Could you check a few things on this model? Use its own coordinates, in mm. Face numbers are marked on the shaded views. A direction names the side the tool comes from. Round coordinates to 2 decimals unless told otherwise and drop trailing zeros. Loops run counter-clockwise (first coordinate to the right, second up) from the corner with the lowest first, then second, coordinate; pieces in that order, holes last. Notation, with made-up numbers: (-23, 4.25) -> (17, 4.25) arc R17 ccw to (17, 30.25) -> close; hole circle Ø8 at (-23.75, -25). An arc over 180 degrees is marked (long way). Put each result on its own line as item: value. Start each with the question number.
1. I'm going to push flat-ended pins straight in: P1, Ø5.5, axis at y = 16, z = -4.5, coming from the +X side; P2, Ø5, axis at x = 6, z = -24.5, coming from the -Y side; P3, Ø8, axis at x = 8, z = -17.5, coming from the +Y side. Where does each tip first touch, or does it pass through?
2. Imagine slicing it at D-D, the plane z = -23.5. Please give me the cut outline in (x, y), and give its area (3 significant figures).
3. Imagine slicing it at C-C, the plane y = 13.5. Please give me the cut outline in (x, z), and give its area (3 significant figures).
4. Which directions (+Z, -Z, +X, -X, +Y, -Y) give clear straight access to the entire face, cutting with the end or side of a thin tool? Please do the marked faces 1, 2 and 3.
5. If we mould it in two halves opening along Y, with no side actions, what happens to the marked faces 4, 5, 6 and 7? For each: pulls with the +Y half, pulls with the -Y half, needs draft (parallel to the pull), parting line crosses it, or undercut.
6. Imagine slicing it at B-B, the plane z = -4. Please give me the cut outline in (x, y), and give its area (3 significant figures).
7. Imagine slicing it at A-A, the plane x = 14.5. Count the separate pieces of the cut face and the enclosed holes in it, and give its area (3 significant figures).
8. I need wall thicknesses on line 1 (Z direction, x = 14.5, y = -0.5); line 2 (X direction, y = -0.5, z = -34); line 3 (Y direction, x = 17, z = -31). Which ranges of each line are inside material? Lowest first, please. Write a range as [from, to].
```python
from build123d import *

# Parameters (mm, degrees)
SALIENTE_EXTRUIR1_DEPTH = 30
REDONDEO1_R             = 1.5
SALIENTE_EXTRUIR2_START = 2.1
SALIENTE_EXTRUIR2_DEPTH = 2.1
SALIENTE_EXTRUIR3_START = 2.1
SALIENTE_EXTRUIR3_DEPTH = 2.1
CROQUIS4_W              = 13.5
CROQUIS4_H              = 8
CROQUIS4_R              = 1.25
SALIENTE_EXTRUIR4_DEPTH = 1
SALIENTE_EXTRUIR5_START = 1
CROQUIS5_W              = 13.5
CROQUIS5_H              = 8
CROQUIS5_R              = 1.25
SALIENTE_EXTRUIR5_DEPTH = 1
REDONDEO2_R             = 1


with BuildPart() as part:
    # Croquis1 → Saliente-Extruir1 (new body)
    with BuildSketch(Plane(origin=(0, 0, 0), x_dir=(1, 0, 0), z_dir=(0, 1, 0))):
        Polygon((0, 0), (9.5, 0), (9.5, 8), (5, 8), (5, 30), (9.5, 30), (9.5, 38), (0, 38), align=None)
    extrude(amount=SALIENTE_EXTRUIR1_DEPTH)

    # Redondeo1
    redondeo1_edges = [part.edges().sort_by_distance(p)[0] for p in [
        (0, 15, -38),
        (9.5, 15, -38),
        (9.5, 15, -30),
        (5, 15, -30),
        (5, 15, -8),
        (9.5, 15, -8),
        (9.5, 15, 0),
        (0, 15, 0),
    ]]
    fillet(redondeo1_edges, radius=REDONDEO1_R)

    # Croquis2 → Saliente-Extruir2 (add)
    with BuildSketch(Plane(origin=(0, 30, 0), x_dir=(1, 0, 0), z_dir=(0, 1, 0)).offset(SALIENTE_EXTRUIR2_START)):
        with BuildLine():
            Line((0, 36.5), (0, 1.5))
            ThreePointArc((0, 1.5), (0.439339828, 0.439339828), (1.5, 0))
            Line((1.5, 0), (8, 0))
            ThreePointArc((8, 0), (9.060660172, 0.439339828), (9.5, 1.5))
            Line((9.5, 1.5), (9.5, 3))
            Line((9.5, 3), (3, 3))
            Line((3, 3), (3, 35))
            Line((3, 35), (9.5, 35))
            Line((9.5, 35), (9.5, 36.5))
            ThreePointArc((9.5, 36.5), (9.060660172, 37.560660172), (8, 38))
            Line((8, 38), (1.5, 38))
            ThreePointArc((1.5, 38), (0.439339828, 37.560660172), (0, 36.5))
        make_face()
    extrude(amount=-SALIENTE_EXTRUIR2_DEPTH)

    # Croquis3 → Saliente-Extruir3 (add)
    with BuildSketch(Plane(origin=(0, 32.1, 0), x_dir=(1, 0, 0), z_dir=(0, 1, 0)).offset(SALIENTE_EXTRUIR3_START)):
        with BuildLine():
            Line((8, 8), (6.5, 8))
            ThreePointArc((6.5, 8), (5.439339828, 8.439339828), (5, 9.5))
            Line((5, 9.5), (5, 28.5))
            ThreePointArc((5, 28.5), (5.439339828, 29.560660172), (6.5, 30))
            Line((6.5, 30), (8, 30))
            ThreePointArc((8, 30), (9.060660172, 30.439339828), (9.5, 31.5))
            Line((9.5, 31.5), (9.5, 36.5))
            ThreePointArc((9.5, 36.5), (9.060660172, 37.560660172), (8, 38))
            Line((8, 38), (1.5, 38))
            ThreePointArc((1.5, 38), (0.439339828, 37.560660172), (0, 36.5))
            Line((0, 36.5), (0, 1.5))
            ThreePointArc((0, 1.5), (0.439339828, 0.439339828), (1.5, 0))
            Line((1.5, 0), (8, 0))
            ThreePointArc((8, 0), (9.060660172, 0.439339828), (9.5, 1.5))
            Line((9.5, 1.5), (9.5, 6.5))
            ThreePointArc((9.5, 6.5), (9.060660172, 7.560660172), (8, 8))
        make_face()
    extrude(amount=-SALIENTE_EXTRUIR3_DEPTH)

    # Croquis4 → Saliente-Extruir4 (add)
    # profile 1 of 2: a face of its own
    with BuildSketch(Plane(origin=(0, 34.2, 0), x_dir=(1, 0, 0), z_dir=(0, 1, 0))):
        with Locations((11, 34)):
            Rectangle(CROQUIS4_W, CROQUIS4_H)
        with Locations(Location((14.5, 34, 0), (0, 0, 270))):
            Circle(CROQUIS4_R, mode=Mode.SUBTRACT)
    # profile 2 of 2: a face of its own
    with BuildSketch(Plane(origin=(0, 34.2, 0), x_dir=(1, 0, 0), z_dir=(0, 1, 0))):
        with Locations((11.5, 4)):
            Rectangle(CROQUIS4_W, CROQUIS4_H)
        with Locations(Location((14.5, 4, 0), (0, 0, 270))):
            Circle(CROQUIS4_R, mode=Mode.SUBTRACT)
    extrude(amount=SALIENTE_EXTRUIR4_DEPTH)

    # Croquis5 → Saliente-Extruir5 (add)
    # profile 1 of 2: a face of its own
    with BuildSketch(Plane.XZ.offset(SALIENTE_EXTRUIR5_START)):
        with Locations((11.5, -4)):
            Rectangle(CROQUIS5_W, CROQUIS5_H)
        with Locations(Location((14.5, -4, 0), (0, 0, 90))):
            Circle(CROQUIS5_R, mode=Mode.SUBTRACT)
    # profile 2 of 2: a face of its own
    with BuildSketch(Plane.XZ.offset(SALIENTE_EXTRUIR5_START)):
        with Locations((11, -34)):
            Rectangle(CROQUIS5_W, CROQUIS5_H)
        with Locations(Location((14.5, -34, 0), (0, 0, 90))):
            Circle(CROQUIS5_R, mode=Mode.SUBTRACT)
    extrude(amount=-SALIENTE_EXTRUIR5_DEPTH)

    # Redondeo2
    redondeo2_edges = [part.edges().sort_by_distance(p)[0] for p in [
        (4.25, 34.7, -38),
        (4.25, 34.7, -30),
        (17.75, 34.7, -30),
        (17.75, 34.7, -38),
        (4.75, 34.7, -8),
        (4.75, 34.7, 0),
        (18.25, 34.7, 0),
        (18.25, 34.7, -8),
        (4.75, -0.5, 0),
        (4.75, -0.5, -8),
        (18.25, -0.5, -8),
        (18.25, -0.5, 0),
        (4.25, -0.5, -30),
        (4.25, -0.5, -38),
        (17.75, -0.5, -38),
        (17.75, -0.5, -30),
    ]]
    fillet(redondeo2_edges, radius=REDONDEO2_R)


solid = part.part
```
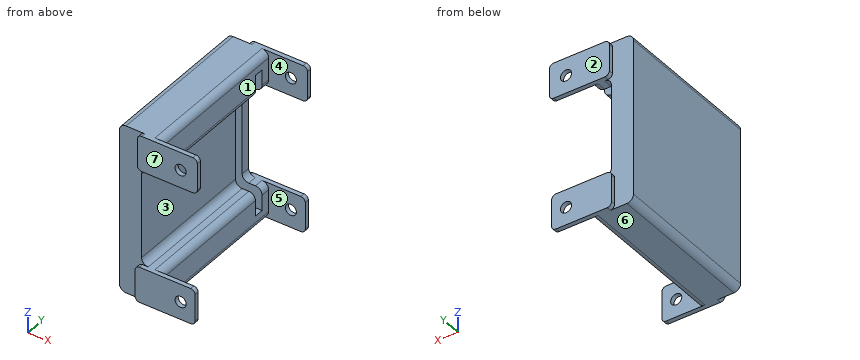
Entries:
1. P1: x = 9.5
1. P2: y = 0
1. P3: y = 34.2
2. outline: (0, 0) -> (5, 0) -> (5, 30) -> (3, 30) -> (3, 32.1) -> (5, 32.1) -> (5, 34.2) -> (0, 34.2) -> close
2. area: 167 mm^2
3. outline: (0, -36.5) arc R1.5 ccw to (1.5, -38) -> (8, -38) arc R1.5 ccw to (9.5, -36.5) -> (9.5, -31.5) arc R1.5 ccw to (8, -30) -> (6.5, -30) arc R1.5 cw to (5, -28.5) -> (5, -9.5) arc R1.5 cw to (6.5, -8) -> (8, -8) arc R1.5 ccw to (9.5, -6.5) -> (9.5, -1.5) arc R1.5 ccw to (8, 0) -> (1.5, 0) arc R1.5 ccw to (0, -1.5) -> close
3. area: 260 mm^2
4. face 1: +Z, -Z, +X
4. face 2: +Z, -Z, +X, -X, +Y
4. face 3: +X, +Y, -Y
5. face 4: undercut
5. face 5: undercut
5. face 6: needs draft
5. face 7: pulls with the -Y half
6. outline: (0, 0) -> (4.75, 0) -> (4.75, -1) -> (13.25, -1) -> (13.25, 0) -> (9.5, 0) -> (9.5, 30) -> (3, 30) -> (3, 32.1) -> (9.5, 32.1) -> (9.5, 34.2) -> (13.25, 34.2) -> (13.25, 35.2) -> (4.75, 35.2) -> (4.75, 34.2) -> (0, 34.2) -> close; (15.75, -1) -> (18.25, -1) -> (18.25, 0) -> (15.75, 0) -> close; (15.75, 34.2) -> (18.25, 34.2) -> (18.25, 35.2) -> (15.75, 35.2) -> close
6. area: 333 mm^2
7. separate pieces: 8
7. enclosed holes: 0
7. area: 22.0 mm^2
8. line 1: [-38, -35.25], [-32.75, -30], [-8, -5.25], [-2.75, 0]
8. line 2: [4.25, 13.25], [15.75, 17.75]
8. line 3: [-1, 0], [34.2, 35.2]
